Could you check a few things on this model? Use its own coordinates, in mm. A direction names the side the tool comes from. Coordinates: 2 decimals unless noted, no trailing zeros. Order: outer loops, then holes, each group sorted by start corner. A loop starts at its lowest first (then second) coordinate and runs counter-clockwise, first axis right, second up. Notation, with made-up numbers: (21, 15) - (79, 15) arc R21 cw to (79, 54) - close; hole circle Ø5 at (22, 79.5). An arc over 180 degrees is marked (long way). Answer as CSV lines item,"result". Start each with the question number.
1. For pin 1 (5 mm diameter, centred on y = 6.5, z = -4, fed in from +X); pin 2 (3 mm diameter, centred on x = 2.5, z = -5, fed in from -Y); pin 3 (8 mm diameter, centred on y = 5.5, z = -21, fed in from -X), each with a flat end and sliding along its axis, tell me the tip position at first contact or that it passes through.
2. I want a section at B-B, the plane y = 9.25. List the corners of the cut face in (x, z) for me.
3. I want a section at A-A, the plane x = 0. List the corners of the cut face in (y, z) for me, and give its area (4 significant figures).
4. For faces 1 (the face through (-2, 5, 0)), 2 (the face through (3.5, 12, -15)), which set-ups out of +Z, -Z, +X, -X, +Y, -Y let a thin tool reach every point of the face, with its end or its side?
5. I want a section at D-D, the plane x = 2.75. List the corners of the cut face in (y, z) for me, and give its area (3 significant figures).
6. I need wall thicknesses on probe 1 along Y at (x, z) = (1.75, -18.5); probe 2 along X at (y, z) = (2.25, 0); probe 3 along Z at (x, y) = (0.5, 11). Which ranges of each line are inside material? Lowest first, please.
7. I want a section at C-C, the plane z = -12.5. List the corners of the cut face in (x, y) for me, and give its area (3 significant figures).
from build123d import *

# Parameters (mm, degrees)
SKETCH_1_R      = 2
EXTRUDE_1_DEPTH = 10
EXTRUDE_2_DEPTH = 5


with BuildPart() as part:
    # Эскиз1 → Бобышка-Вытянуть1 (new body)
    with BuildSketch(Plane(origin=(0, 0, 0), x_dir=(1, 0, 0), z_dir=(0, 1, 0))):
        with Locations(Location((0, 0, 0), (0, 0, 270))):
            Circle(SKETCH_1_R)
    extrude(amount=EXTRUDE_1_DEPTH)

    # Эскиз2 → Бобышка-Вытянуть2 (add)
    with BuildSketch(Plane(origin=(0, 10, 0), x_dir=(1, 0, 0), z_dir=(0, 1, 0))):
        with BuildLine():
            Line((-3.5, 0), (-3.5, 30))
            Line((-3.5, 30), (3.5, 30))
            Line((3.5, 30), (3.5, 0))
            ThreePointArc((3.5, 0), (0, -3.5), (-3.5, 0))
        make_face()
    extrude(amount=EXTRUDE_2_DEPTH)


solid = part.part
Solved:
1,pin 1,"stops at x = 1.32"
1,pin 2,"stops at y = 10"
1,pin 3,"passes through"
2,outline,"circle Ø4 at (0, 0)"
3,outline,"(0, -2) - (10, -2) - (10, -30) - (15, -30) - (15, 3.5) - (10, 3.5) - (10, 2) - (0, 2) - close"
3,area,"207.5 mm2"
4,face 1,"-Y"
4,face 2,"+Z, -Z, +X, +Y, -Y"
5,outline,"(10, -30) - (15, -30) - (15, 2.17) - (10, 2.17) - close"
5,area,"161 mm2"
6,probe 1,"y = 10 to 15"
6,probe 2,"x = -2 to 2"
6,probe 3,"z = -30 to 3.46"
7,outline,"(-3.5, 10) - (3.5, 10) - (3.5, 15) - (-3.5, 15) - close"
7,area,"35.0 mm2"
